```python
from build123d import *

# Parameters (mm, degrees)
SKETCH1_R           = 2.286
SKETCH1_W           = 6.477
SKETCH1_H           = 6.477
BOSS_EXTRUDE1_DEPTH = 4.7625


with BuildPart() as part:
    # Sketch1 → Boss-Extrude1 (new body)
    with BuildSketch(Plane.XY):
        with BuildLine():
            Line((-6.235543901, 1.200205089), (3.330554168, 50.899898088))
            ThreePointArc((3.330554168, 50.899898088), (3.347215179, 50.989952859), (3.362575674, 51.080238551))
            Line((3.362575674, 51.080238551), (12.782434592, 108.969864627))
            ThreePointArc((12.782434592, 108.969864627), (19.731964071, 114.263273715), (25.390778308, 107.607902862))
            Line((25.390778308, 107.607902862), (22.211167462, 48.67374279))
            ThreePointArc((22.211167462, 48.67374279), (22.06323721, 47.438914255), (21.755683067, 46.233885077))
            Line((21.755683067, 46.233885077), (6.037122044, -1.968668947))
            ThreePointArc((6.037122044, -1.968668947), (-1.587540069, -6.148350716), (-6.235543901, 1.200205089))
        make_face()
        with Locations(Location((0, 0, 0), (0, 0, 180))):
            Circle(SKETCH1_R, mode=Mode.SUBTRACT)
        with Locations(Location((19.05, 107.95, 0), (0, 0, 180))):
            Circle(SKETCH1_R, mode=Mode.SUBTRACT)
        with Locations((12.7, 49.186888497)):
            Rectangle(SKETCH1_W, SKETCH1_H, mode=Mode.SUBTRACT)
    extrude(amount=BOSS_EXTRUDE1_DEPTH)


solid = part.part
```
Can you work these out from the model? Positions are in its coordinate system, mm. A direction names the side the tool comes from. Give positions to 0.01 mm unless a question says otherwise; leave off trailing zeros. Write each loop counter-clockwise with the first axis right and the second up, starting at its lowest first coordinate (ties: lowest second). Pieces come first, ordered by that corner, then holes. Notation, with made-up numbers: (75, -9) - (128, -9) arc R14 cw to (128, 0) - close; hole circle Ø10 at (10.5, 20). An arc over 180 degrees is marked (long way). Write item = value, one per line. Start each with the question number.
1. Imagine slicing it at D-D (y = 12.5). Please give me the cut outline in (x, z), and give its area (3 significant figures).
2. Imagine slicing it at A-A (z = 2.55). Count the separate pieces of the cut face and the enclosed holes in it, and give its area (3 significant figures).
3. Please list where these lines run through material, in increasing order: line 1 (X direction, y = 21, z = 1.95); line 2 (X direction, y = 108, z = 2.3); line 3 (X direction, y = 5, z = 3).
4. Imagine slicing it at B-B (x = 0). Please give me the cut outline in (y, z), and give its area (3 significant figures).
5. For pin 1 (4 mm diameter, centred on x = 0, y = 0, fed in from +Z); pin 2 (2.5 mm diameter, centred on y = 50.5, z = 2.5, fed in from +X); pin 3 (1.4 mm diameter, centred on y = 48.5, z = 2, fed in from -X), each with a flat end and sliding along its axis, tell me the tip position at first contact or that it passes through.
6. On a 3-axis mill with a long thin cutter (end or side, diameter ignored), from which of +Z, -Z, +X, -X, +Y, -Y can I reach the whole of each face in a straight line? I mean faces 5 (the face through (10, 55, 0)), 6 (the face through (13, 45.948, 2)). Say none if no direction works.
7. Imagine slicing it at C-C (y = 0). Please give me the cut outline in (x, z), and give its area (3 significant figures).
8. Thinking about a two-plate mould opening in Y: for faces 1 (the face through (13, 52.425, 2)), 2 (the face through (8.007, 79.62, 2.348)), 3 (the face through (14.006, 22.47, 2.348)), 4 (the face through (10, 55, 4.762)), which applies, released by +Y, released by -Y, zero draft, split by the parting line, or undercut?
Worked answers:
q1.outline = (-4.06, 0) - (10.76, 0) - (10.76, 4.76) - (-4.06, 4.76) - close
q1.area = 70.6 mm2
q2.separate_pieces = 1
q2.enclosed_holes = 3
q2.area = 1,800 mm2
q3.line_1 = -2.42 to 13.53
q3.line_2 = 12.62 to 16.76, 21.34 to 25.4
q3.line_3 = -5.5 to 8.31
q4.outline = (-6.35, 0) - (-2.29, 0) - (-2.29, 4.76) - (-6.35, 4.76) - close; (2.29, 0) - (33.6, 0) - (33.6, 4.76) - (2.29, 4.76) - close
q4.area = 168 mm2
q5.pin_1 = through
q5.pin_2 = 22.38
q5.pin_3 = 2.73
q6.face_5 = -Z, +X, -X, +Y, -Y
q6.face_6 = +Z, -Z
q7.outline = (-6.35, 0) - (-2.29, 0) - (-2.29, 4.76) - (-6.35, 4.76) - close; (2.29, 0) - (6.68, 0) - (6.68, 4.76) - (2.29, 4.76) - close
q7.area = 40.3 mm2
q8.face_1 = undercut
q8.face_2 = released by +Y
q8.face_3 = released by -Y
q8.face_4 = zero draft
